Design review of the part built by this model. Coordinates are the model's own, in mm. A direction names the side the tool comes from. Round coordinates to 2 decimals unless told otherwise and drop trailing zeros. Loops run counter-clockwise (first coordinate to the right, second up) from the corner with the lowest first, then second, coordinate; pieces in that order, holes last. Notation, with made-up numbers: (-28.5, 41.25) - (29.5, 41.25) arc R21 cw to (29.5, 50.25) - close; hole circle Ø5 at (-33, 33). An arc over 180 degrees is marked (long way). One line per question, with ' | ' between items. Start each with the question number.
from build123d import *

# Parameters (mm, degrees)
SKETCH_1_R          = 15
EXTRUDE_1_DEPTH     = 8
SKETCH_1_3_R        = 14.25
EXTRUDE_2_DEPTH     = 18
SKETCH_2_R          = 3
CUT_EXTRUDE_1_DEPTH = 34.555923471


with BuildPart() as part:
    # Sketch 1 → Extrude 1 (new body)
    with BuildSketch(Plane(origin=(0, 0, 0), x_dir=(1, 0, 0), z_dir=(0, 1, 0))):
        with Locations(Location((0, 0, 0), (0, 0, 270))):
            Circle(SKETCH_1_R)
    extrude(amount=EXTRUDE_1_DEPTH)

    # Sketch 1_3 → Extrude 2 (add)
    with BuildSketch(Plane(origin=(0, 0, 0), x_dir=(1, 0, 0), z_dir=(0, 1, 0))):
        with Locations(Location((0, 0, 0), (0, 0, 270))):
            Circle(SKETCH_1_3_R)
    extrude(amount=-EXTRUDE_2_DEPTH)

    # Sketch 2 → Cut-Extrude 1 (cut, through all)
    with BuildSketch(Plane(origin=(0, 8, 0), x_dir=(1, 0, 0), z_dir=(0, 1, 0))):
        with Locations(Location((0, 0, 0), (0, 0, 270))):
            Circle(SKETCH_2_R)
        with Locations(Location((0, 8, 0), (0, 0, 270))):
            Circle(SKETCH_2_R)
        with Locations(Location((6.92820323, -4, 0), (0, 0, 270))):
            Circle(SKETCH_2_R)
        with Locations(Location((-6.92820323, -4, 0), (0, 0, 270))):
            Circle(SKETCH_2_R)
    extrude(amount=-CUT_EXTRUDE_1_DEPTH, mode=Mode.SUBTRACT)


solid = part.part
1. Machinability: for faces 1 (the face through (0.66, 3.944, -14.985)), 2 (the face through (-13.91, -8.87, -3.09)), which of the approach directions +Z, -Z, +X, -X, +Y, -Y give a long, thin tool a straight path to every point of the face, cutting with its end or side? Answer none if there is none.
2. To check wall thickness, follow line 1 along Z through (x, y) = (2.5, -12.5); line 2 along X through (y, z) = (-1, 2.5); line 3 along X through (y, z) = (-1.75, 0). State the ranges of each line that lie inside material, in increasing order.
3. Clearance check with flat-ended pins moving along their axes: P1, Ø1.5, axis at x = 2.5, y = -0.5, coming from the +Z side; P2, Ø1, axis at y = -1.5, z = -11.5, coming from the +X side; P3, Ø8, axis at y = 2, z = 1.5, coming from the +X side; P4, Ø5, axis at y = -13.5, z = -7.5, coming from the -X side. State where each tip first meets the part, or that it passes through.
4. Take a section at A-A, the plane x = 0. Give the boundary of the cut face in (y, z).
5. Take a section at B-B, the plane z = 0. Give the boundary of the cut face in (x, y).
6. Take a section at C-C, the plane z = 6.5. Give the boundary of the cut face in (x, y).
7. Take a section at D-D, the plane x = 5.25. Give the boundary of the cut face in (y, z).
Answer list:
1) face 1: +Y, -Y | face 2: -Y
2) line 1: z = -14.03 to -9.66, -6.34 to -1.66, 1.66 to 14.03 | line 2: x = -14.03 to -9.53, -4.33 to -1.66, 1.66 to 4.33, 9.53 to 14.03 | line 3: x = -14.25 to -3, 3 to 14.25
3) P1: stops at z = 14.87 | P2: stops at x = 9.06 | P3: stops at x = 15 | P4: stops at x = -13.34
4) outline: (-18, -14.25) - (0, -14.25) - (0, -15) - (8, -15) - (8, -11) - (-18, -11) - close; (-18, -5) - (8, -5) - (8, -3) - (-18, -3) - close; (-18, 3) - (8, 3) - (8, 15) - (0, 15) - (0, 14.25) - (-18, 14.25) - close
5) outline: (-15, 0) - (-14.25, 0) - (-14.25, -18) - (-3, -18) - (-3, 8) - (-15, 8) - close; (3, -18) - (14.25, -18) - (14.25, 0) - (15, 0) - (15, 8) - (3, 8) - close
6) outline: (-13.52, 0) - (-12.68, 0) - (-12.68, -18) - (-8.59, -18) - (-8.59, 8) - (-13.52, 8) - close; (-5.27, -18) - (5.27, -18) - (5.27, 8) - (-5.27, 8) - close; (8.59, -18) - (12.68, -18) - (12.68, 0) - (13.52, 0) - (13.52, 8) - (8.59, 8) - close
7) outline: (-18, -13.25) - (0, -13.25) - (0, -14.05) - (8, -14.05) - (8, 1.51) - (-18, 1.51) - close; (-18, 6.49) - (8, 6.49) - (8, 14.05) - (0, 14.05) - (0, 13.25) - (-18, 13.25) - close
